Source: three-view drawing plus pictorial views. Frame: mm from the lowest corner of the part. A direction names the side the tool comes from. Give positions to 0.01 mm unless a question says otherwise; leave off trailing zeros. Write each loop counter-clockwise with the first axis right and the second up, starting at its lowest first coordinate (ties: lowest second). Pieces come first, ordered by that corner, then holes. Notation, with made-up numbers: (-5, 33.25) -> (27, 33.25) arc R12 ccw to (27, 53.25) -> close; hole circle Ø11 at (30.5, 11.25). An arc over 180 degrees is marked (long way). Write item = value, one per line.
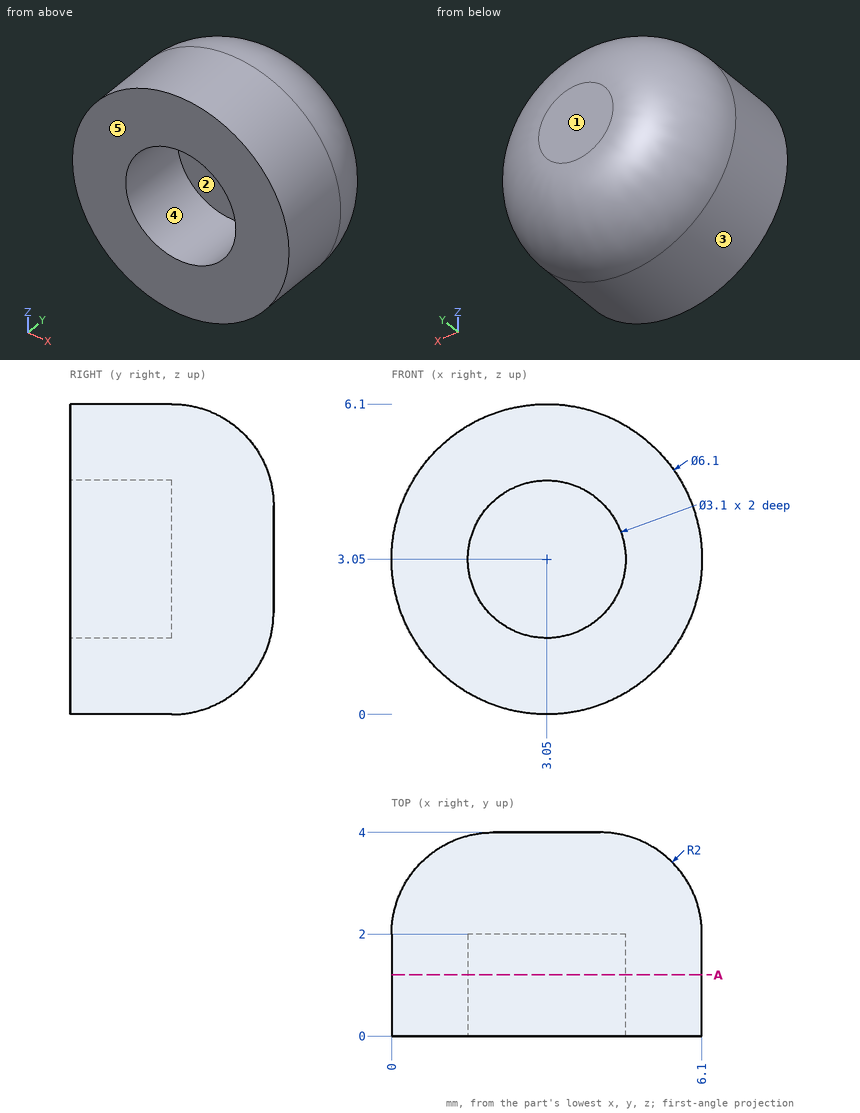
1) Draft query along X for the marked faces 3, 4 and 5. Return one class per face: pulls with the +X half, pulls with the -X half, needs draft (parallel to the pull), parting line crosses it, or undercut.
Computed:
face_3 = parting line crosses it
face_4 = undercut
face_5 = needs draft
2) Material intervals for L1, parallel to Z at x = 3.05, y = 1.05; L2, parallel to Y at x = 3.75, z = 3; L3, parallel to X at y = 1.5, z = 3.5, sorted ascending.
Computed:
L1 = 0 to 1.5, 4.6 to 6.1
L2 = 2 to 4
L3 = 0.03 to 1.57, 4.53 to 6.07
3) Cut plane A-A (y = 1.2). Return the cut outline in (x, z), then the cut area to 3 significant figures.
Computed:
outline = circle Ø6.1 at (3.05, 3.05); hole circle Ø3.1 at (3.05, 3.05)
area = 21.7 mm²
4) Contact query for flat-ended pins moving along their axis: pin 1 (1 mm diameter, centred on y = 1, z = 2, fed in from +X); pin 2 (2 mm diameter, centred on y = 3, z = 2, fed in from +X). Output: stop coordinate, or through.
Computed:
pin_1 = 6.05
pin_2 = 6.06
5) Access query for the marked faces 1 and 2. Directions: +Z, -Z, +X, -X, +Y, -Y. A direction counts if a zero-diameter tool reaches every point of the face in a straight line with its end or side. Return the directions, or none.
Computed:
face_1 = +Z, -Z, +X, -X, +Y
face_2 = -Y
